Design review of the part built by this model. Coordinates are the model's own, in mm. Face numbers are marked on the shaded views. Coordinates: 2 decimals unless noted, no trailing zeros. Loops run counter-clockwise (first coordinate to the right, second up) from the corner with the lowest first, then second, coordinate; pieces in that order, holes last. Notation, with made-up numbers: (70.25, 39) -> (113.25, 39) arc R18 cw to (113.25, 60) -> close; hole circle Ø1 at (-1.5, -25.5). An arc over 180 degrees is marked (long way). Answer in a Markdown table with one row per item.
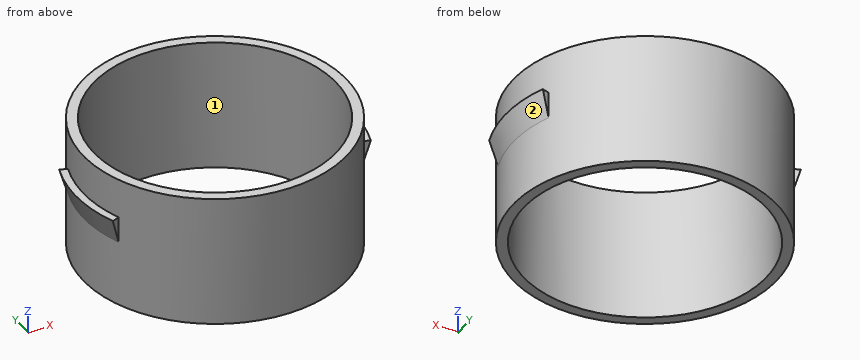
Solid Edge part; units mm, degrees
sketch "Sketch1" plane through (0, 0, 0) normal (0, 0, 1) x (1, 0, 0)
  circle A0 centre (0, 0) radius 25
  circle A1 centre (0, 0) radius 23
extrude "Protrusion1" add sketch "Sketch1" along normal blind 25
sketch "Sketch2" plane through (0, 0, 0) normal (0, -1, 0) x (1, 0, 0)
  line L0 (26.5, 12.5) -> (25, 7.5023)
  line L1 (25, 7.5023) -> (25, 12.5)
  line L2 (25, 12.5) -> (26.5, 12.5)
revolve "RevolvedProtrusion_1" add sketch "Sketch2" angle 40 mid plane about axis through (0, 0, 0) along (0, 0, 1)
mirror "Mirror1" about plane through (0, 0, 0) normal (1, 0, 0) of "RevolvedProtrusion_1"
sketch "Sketch3" plane through (0, 0, 0) normal (0, 0, 1) x (1, 0, 0)
  circle A0 centre (0, 0) radius 25
  circle A1 centre (0, 0) radius 23
extrude "Protrusion2" add sketch "Sketch3" against normal blind 5
sketch "Sketch4" plane through (0, 0, 25) normal (0, 0, 1) x (1, 0, 0)
  circle A0 centre (0, 0) radius 25
extrude "ExtrudedCutout_1" cut sketch "Sketch4" against normal blind 5
(1) To check wall thickness, follow probe 1 along X at (y, z) = (0, 6.75); probe 2 along Y at (x, z) = (-19, 1). State the ranges of each line that lie inside material, in increasing order.
Evaluation:
| item | result |
|---|---|
| probe 1 | x = -25 to -23, 23 to 25 |
| probe 2 | y = -16.25 to -12.96, 12.96 to 16.25 |
(2) Take a section at B-B on y = -16. Give the boundary of the cut face in (x, z).
Evaluation:
| item | result |
|---|---|
| outline | (-19.21, -5) -> (-16.52, -5) -> (-16.52, 20) -> (-19.21, 20) -> close; (16.52, -5) -> (19.21, -5) -> (19.21, 20) -> (16.52, 20) -> close |
(3) Take a section at D-D on y = 0. Give the boundary of the cut face in (x, z).
Evaluation:
| item | result |
|---|---|
| outline | (-26.5, 12.5) -> (-25, 7.5) -> (-25, -5) -> (-23, -5) -> (-23, 20) -> (-25, 20) -> (-25, 12.5) -> close; (23, -5) -> (25, -5) -> (25, 7.5) -> (26.5, 12.5) -> (25, 12.5) -> (25, 20) -> (23, 20) -> close |
(4) Take a section at A-A on x = 20. Give the boundary of the cut face in (y, z).
Evaluation:
| item | result |
|---|---|
| outline | (-15, -5) -> (-11.36, -5) -> (-11.36, 20) -> (-15, 20) -> close; (11.36, -5) -> (15, -5) -> (15, 20) -> (11.36, 20) -> close |
(5) Take a section at C-C on z = 8.5. Give the boundary of the cut face in (x, y).
Evaluation:
| item | result |
|---|---|
| outline | (-23.77, -8.65) -> (-23.49, -8.55) arc R25 ccw to (23.49, -8.55) -> (23.77, -8.65) arc R25.3 ccw to (23.77, 8.65) -> (23.49, 8.55) arc R25 ccw to (-23.49, 8.55) -> (-23.77, 8.65) arc R25.3 ccw to start; hole circle Ø46 at (0, 0) |
(6) For pin 1 (5 mm diameter, centred on y = -13.5, z = 5, fed in from -X); pin 2 (3 mm diameter, centred on x = 11, z = 4.5, fed in from +Y); pin 3 (0.9 mm diameter, centred on x = -25.5, y = 3.5, fed in from +Z), all flat-tipped, find the tip position at first contact; note any pin that passes through.
Evaluation:
| item | result |
|---|---|
| pin 1 | stops at x = -22.45 |
| pin 2 | stops at y = 23.12 |
| pin 3 | stops at z = 12.5 |
(7) Draft analysis for pull direction Y (two halves, no side actions). For the marked faces 1 and 2, state which applies: pulls with the +Y half, pulls with the -Y half, needs draft (parallel to the pull), parting line crosses it, or undercut.
Evaluation:
| item | result |
|---|---|
| face 1 | undercut |
| face 2 | parting line crosses it |
